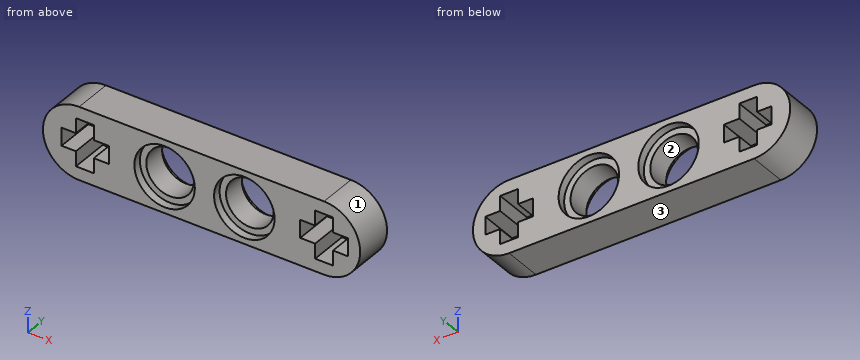
from build123d import *

# Parameters (mm, degrees)
SKETCH1_R           = 2.4
BOSS_EXTRUDE1_DEPTH = 3.9
SKETCH2_R           = 3.05
CUT_EXTRUDE1_DEPTH  = 0.8
SKETCH3_R           = 3.05
CUT_EXTRUDE2_DEPTH  = 0.8


with BuildPart() as part:
    # Sketch1 → Boss-Extrude1 (new body)
    with BuildSketch(Plane(origin=(0, 0, 0), x_dir=(1, 0, 0), z_dir=(0, 1, 0))):
        with BuildLine():
            Line((-12.665, 3.65), (12.035, 3.65))
            ThreePointArc((12.035, 3.65), (15.685, 0), (12.035, -3.65))
            Line((12.035, -3.65), (-12.665, -3.65))
            ThreePointArc((-12.665, -3.65), (-16.315, 0), (-12.665, 3.65))
        make_face()
        with Locations((-4.045, 0.018008222)):
            Circle(SKETCH1_R, mode=Mode.SUBTRACT)
        with Locations((3.995, 0.008270612)):
            Circle(SKETCH1_R, mode=Mode.SUBTRACT)
        Polygon((11.135, 2.4), (11.135, 0.9), (9.635, 0.9), (9.635, -0.9), (11.135, -0.9), (11.135, -2.4), (12.935, -2.4), (12.935, -0.9), (14.435, -0.9), (14.435, 0.9), (12.935, 0.9), (12.935, 2.4), align=None, mode=Mode.SUBTRACT)
        Polygon((-12.985, 2.401087844), (-12.985, 0.901087844), (-14.433060202, 0.901087844), (-14.433060202, -0.898912156), (-12.985, -0.898912156), (-12.985, -2.398912156), (-11.185, -2.398912156), (-11.185, -0.898912156), (-9.633060202, -0.898912156), (-9.633060202, 0.901087844), (-11.185, 0.901087844), (-11.185, 2.401087844), align=None, mode=Mode.SUBTRACT)
    extrude(amount=BOSS_EXTRUDE1_DEPTH)

    # Sketch2 → Cut-Extrude1 (cut)
    with BuildSketch(Plane(origin=(0, 3.9, 0), x_dir=(1, 0, 0), z_dir=(0, 1, 0))):
        with Locations((-4.045, 0.018008222)):
            Circle(SKETCH2_R)
        with Locations((3.995, 0.008270612)):
            Circle(SKETCH2_R)
    extrude(amount=-CUT_EXTRUDE1_DEPTH, mode=Mode.SUBTRACT)

    # Sketch3 → Cut-Extrude2 (cut)
    with BuildSketch(Plane.XZ):
        with Locations((3.995, -0.008270612)):
            Circle(SKETCH3_R)
        with Locations((-4.045, -0.018008222)):
            Circle(SKETCH3_R)
    extrude(amount=-CUT_EXTRUDE2_DEPTH, mode=Mode.SUBTRACT)


solid = part.part
Check sheet for the modelled part. Datum: model origin and axes. Units: mm. Face numbers are marked on the shaded views. Round coordinates to 2 decimals unless told otherwise and drop trailing zeros. Order: outer loops, then holes, each group sorted by start corner. A loop starts at its lowest first (then second) coordinate and runs counter-clockwise, first axis right, second up.
(1) Cross-section at B-B, the plane y = 3.5. State how many separate pieces and enclosed holes the cut face has, and give its area (3 significant figures).
(2) Cross-section at A-A, the plane x = -10. Enter the section's corners in (y, z).
(3) Scan lines: probe 1 along X at (y, z) = (1.05, 0.5) (3 decimals); probe 2 along X at (y, z) = (0.4, -1.25) (3 decimals); probe 3 along Z at (x, y) = (-12.5, 2.1). Record each from-to range of solid material in increasing order.
(4) Draft check along X on the marked faces 1, 2 and 3. Enter one of: pulls with the +X half, pulls with the -X half, needs draft (parallel to the pull), parting line crosses it, or undercut.
(5) Go/stop test with flat-tipped pins: P1, Ø1, axis at x = -2, z = -0.5, coming from the -Y side; P2, Ø1.6, axis at y = 2.5, z = -1.5, coming from the -X side; P3, Ø3.5, axis at x = -4.04, z = -0.02, coming from the -Y side; P4, Ø1.2, axis at y = 1, z = -2, coming from the +X side. Record where each tip stops, or that it passes through.
Check sheet entries:
1. separate pieces: 1
1. enclosed holes: 4
1. area: 136 mm2
2. outline: (0, -3.65) - (3.9, -3.65) - (3.9, -0.9) - (0, -0.9) - close; (0, 0.9) - (3.9, 0.9) - (3.9, 3.65) - (0, 3.65) - close
3. probe 1: x = -16.281 to -14.433, -9.633 to -6.388, -1.702 to 1.649, 6.341 to 9.635, 14.435 to 15.651
3. probe 2: x = -16.094 to -12.985, -11.185 to -6.835, -1.255 to 1.209, 6.781 to 11.135, 12.935 to 15.464
3. probe 3: z = -3.65 to -2.4, 2.4 to 3.65
4. face 1: pulls with the +X half
4. face 2: undercut
4. face 3: needs draft
5. P1: stops at y = 0.8
5. P2: stops at x = -16.25
5. P3: passes through
5. P4: stops at x = 15.41
